from build123d import *

# Parameters (mm, degrees)
F1_DEPTH  = 505
F2_DEPTH  = 500.5
F4_DEPTH  = 10
F5_DEPTH  = 10
F7_DEPTH  = 3.5
F8_W      = 10
F8_H      = 10
F10_DEPTH = 0.5
F11_DEPTH = 3.5
F12_W     = 3
F12_H     = 158.2
F12_H_2   = 149.0364306936
F12_H_3   = 168.1512820513
F13_DEPTH = 3
F14_W     = 3
F14_H     = 180.2518238002
F14_H_2   = 163.2489754916
F14_H_3   = 161.2561033061
F15_DEPTH = 3
F16_DEPTH = 40
F17_W     = 5.5675039161
F17_H     = 3.688506484
F18_DEPTH = 25
F19_DEPTH = 25


with BuildPart() as f1:
    # F0 (on Front) → F1 (new body)
    with BuildSketch(Plane.XZ):
        Polygon((5, 0), (0, 0), (-5, 0), (-5, -200), (5, -200), align=None)
    extrude(amount=F1_DEPTH)

    # F0 (on Front) → F2 (join)
    with BuildSketch(Plane.XZ):
        Polygon((5, 0), (0, 0), (-5, 0), (-5, -200), (5, -200), align=None)
    extrude(amount=F2_DEPTH)

    # F3 (on face) → F4 (cut, through all)
    with BuildSketch(Plane(origin=(-5, 0, 0), x_dir=(0, -1, 0), z_dir=(-1, 0, 0))):
        Polygon((328.8512820513, -65.3208171387), (328.8512820513, -5), (179.8148513577, -5), align=None)
        Polygon((173.1512820513, -128.1396039604), (325.4411393395, -69.334609562), (173.1512820513, -7.6970046434), align=None)
        Polygon((168.1512820513, -5), (0, -5), (0, -195), (168.1512820513, -130.0702970297), align=None)
        Polygon((333.8512820513, -66.0871287129), (492.0512820513, -5), (333.8512820513, -5), align=None)
    extrude(amount=-F4_DEPTH, mode=Mode.SUBTRACT)

    # F3 (on face) → F5 (cut, through all)
    with BuildSketch(Plane(origin=(-5, 0, 0), x_dir=(0, -1, 0), z_dir=(-1, 0, 0))):
        Polygon((505, -200), (505, -5), (331.3512820513, -72.0524752475), (0, -200), align=None)
    extrude(amount=-F5_DEPTH, mode=Mode.SUBTRACT)

    # F6 (on face) → F7 (cut)
    with BuildSketch(Plane(origin=(-5, 0, 0), x_dir=(0, -1, 0), z_dir=(-1, 0, 0))):
        Polygon((179.8148513577, -5), (168.1512820513, -5), (168.1512820513, -130.0702970297), (173.1512820513, -128.1396039604), (173.1512820513, -7.6970046434), (325.4411393395, -69.334609562), (333.8512820513, -66.0871287129), (333.8512820513, -5), (328.8512820513, -5), (328.8512820513, -65.3208171387), align=None)
    extrude(amount=-F7_DEPTH, mode=Mode.SUBTRACT)

    # F8 (on face) → F10 (join)
    with BuildSketch(Plane.XY):
        with Locations((0, -500)):
            Rectangle(F8_W, F8_H)
    extrude(amount=F10_DEPTH)

    # F9 (on face) → F11 (cut)
    with BuildSketch(Plane.YZ.offset(5)):
        Polygon((-173.1512820513, -7.6970046434), (-173.1512820513, -128.1396039604), (-168.1512820513, -130.0702970297), (-168.1512820513, -5), (-179.8148513577, -5), (-328.8512820513, -65.3208171387), (-328.8512820513, -5), (-333.8512820513, -5), (-333.8512820513, -66.0871287129), (-325.4411393395, -69.334609562), align=None)
    extrude(amount=-F11_DEPTH, mode=Mode.SUBTRACT)

    # F12 (on face) → F13 (join)
    with BuildSketch(Plane(origin=(0, 0, -5), x_dir=(1, 0, 0), z_dir=(0, 0, -1))):
        with Locations((0, 412.9512820513)):
            Rectangle(F12_W, F12_H)
        with Locations((0, 254.3330667045)):
            Rectangle(F12_W, F12_H_2)
        with Locations((0, 84.0756410256)):
            Rectangle(F12_W, F12_H_3)
    extrude(amount=F13_DEPTH)

    # F14 (on face) → F15 (join)
    with BuildSketch(Plane(origin=(0, -65.5267872377, -169.6975772053), x_dir=(1, 0, 0), z_dir=(0, 0.3602166214, 0.9328686862))):
        with Locations((0, -19.8836707273)):
            Rectangle(F14_W, F14_H)
        with Locations((0, -196.9938815385)):
            Rectangle(F14_W, F14_H_2)
        with Locations((0, -368.2617762991)):
            Rectangle(F14_W, F14_H_3)
    extrude(amount=F15_DEPTH)

    # F16 (add): a face of the model
    f16_faces = [f1.faces().sort_by_distance(p)[0] for p in [
        (0, -167.6109571192, -128.6709940004),
    ]]
    extrude(f16_faces, amount=F16_DEPTH)

    # F17 (on face) → F18 (cut)
    with BuildSketch(Plane(origin=(0, 0, 0), x_dir=(-1, 0, 0), z_dir=(0, 1, 0))):
        with Locations((-0.283751958, -193.155746758)):
            Rectangle(F17_W, F17_H)
    extrude(amount=F18_DEPTH, mode=Mode.SUBTRACT)

    # F19 (cut): a face of the model
    f19_faces = [f1.faces().sort_by_distance(p)[0] for p in [
        (-1.5, -84.0756410256, -7.4725396089),
    ]]
    extrude(f19_faces, amount=-F19_DEPTH, mode=Mode.SUBTRACT)


solid = f1.part
For this review, take the finished solid that the model builds, in its own axes (mm). A direction names the side the tool comes from. Round coordinates to 2 decimals unless told otherwise and drop trailing zeros. Write each loop counter-clockwise with the first axis right and the second up, starting at its lowest first coordinate (ties: lowest second). Pieces come first, ordered by that corner, then holes. Notation, with made-up numbers: M -8.75,-19 L 48.25,-19 A14 cw 48.25,-1 Z; hole C 59,63 d6. An arc over 180 degrees is marked long. Write item = value, one per line. Start each with the question number.
(1) For faces 1 (the face through (0, -244, 0)), 2 (the face through (5, -272, -4)), list the 3-axis set-ups (+Z, -Z, +X, -X, +Y, -Y) from which the entire face can be reached by the end or side of a thin tool; tool diameter is ignored.
(2) We need section B-B (x = 0). Give the boundary of the cut face in (y, z), then the cut area to 3 significant figures.
(3) The part is to be moulded in two halves that separate along Z. For faces 3 (the face through (0, -249, -5)), 4 (the face through (0, -500, 0.5)), 5 (the face through (-0.07, -256.035, -101.135)), say which applies: +Z half, -Z half, draft (parallel to the pull), parting line (faces both ways), or undercut.
(4) For line 1 along Z through (x, y) = (2.5, -355); line 2 along Z through (x, y) = (0.5, -214), list the stretches that pass through material, from the lowest coordinate up.
(5) We need section A-A (y = -192). Give the boundary of the cut face in (x, z), then the cut area to 4 significant figures.
(6) Clearance check with a flat-ended pin moving along its axis: pin 1 Ø3 at (x, y) = (1, -158) entering from +Z. State where the tip first meets the part, or that it passes through.
(7) We need section C-C (z = -113). Give the boundary of the cut face in (x, y).
Results found:
q1.face_1 = +Z, +X, -X, +Y
q1.face_2 = +Z, -Z, +X, +Y, -Y
q2.outline = M -505,-5 L 0,-200 L 0,-195 L -492.05,-5 L 0,-5 L 0,0 L -495,0 L -495,0.5 L -505,0.5 Z
q2.area = 5,020 mm²
q3.face_3 = undercut
q3.face_4 = +Z half
q3.face_5 = -Z half
q4.line_1 = -62.92 to -57.92, -5 to 0
q4.line_2 = -117.37 to -112.37, -5 to 0
q5.outline = M -5,-125.86 L 5,-125.86 L 5,-120.86 L -5,-120.86 Z; M -5,-5 L 5,-5 L 5,0 L -5,0 Z
q5.area = 100.0 mm²
q6.pin_1 = 0
q7.outline = M -5,-225.31 L 5,-225.31 L 5,-212.36 L -5,-212.36 Z
